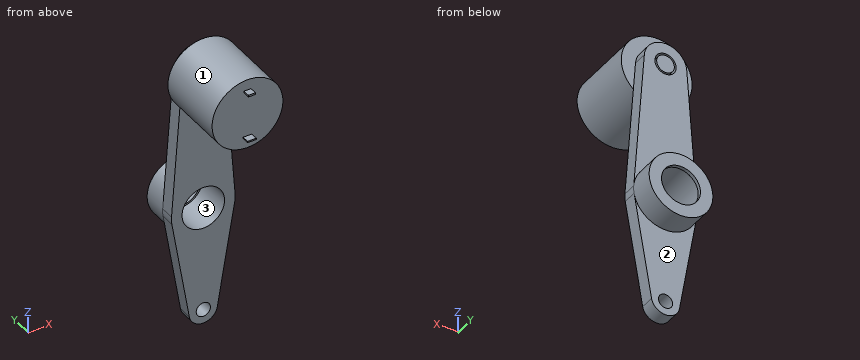
from build123d import *

# Parameters (mm, degrees)
EXTRUDE_1_DEPTH       = 4
SKETCH_3_R            = 9
EXTRUDE_2_DEPTH       = 7
SKETCH_4_R            = 3
CUT_EXTRUDE_1_DEPTH   = 48.391982444
SKETCH_5_R            = 6
CUT_EXTRUDE_2_DEPTH   = 10
SKETCH_7_R            = 5.5
CUT_EXTRUDE_3_DEPTH   = 49.145612469
HOLE_WIZARD_4_0_4_1_D = 4
SCALE1_SCALE          = 2
SKETCH1_R             = 20
EXTRUDE1_DEPTH        = 40
SKETCH2_R             = 5
EXTRUDE2_DEPTH        = 8
SKETCH3_W             = 4
SKETCH3_H             = 1
SKETCH3_W_2           = 4.944968004
SKETCH3_H_2           = 0.773994992
EXTRUDE3_DEPTH        = 4


with BuildPart() as part:
    # 草图1 → 凸台-拉伸1 (new body)
    with BuildSketch(Plane(origin=(0, 0, 0), x_dir=(1, 0, 0), z_dir=(0, 1, 0))):
        with BuildLine():
            Line((-8.974651804, -0.675), (-5.983101203, -40.45))
            ThreePointArc((-5.983101203, -40.45), (0, -46), (5.983101203, -40.45))
            Line((5.983101203, -40.45), (8.974651804, -0.675))
            ThreePointArc((8.974651804, -0.675), (8.990401386, 0.415551353), (8.874119675, 1.5))
            Line((8.874119675, 1.5), (3.944053189, 30.666666667))
            ThreePointArc((3.944053189, 30.666666667), (0, 34), (-3.944053189, 30.666666667))
            Line((-3.944053189, 30.666666667), (-8.874119675, 1.5))
            ThreePointArc((-8.874119675, 1.5), (-8.990401386, 0.415551353), (-8.974651804, -0.675))
        make_face()
    extrude(amount=EXTRUDE_1_DEPTH)

    # 草图3 → 凸台-拉伸2 (add)
    with BuildSketch(Plane(origin=(0, 4, 0), x_dir=(1, 0, 0), z_dir=(0, 1, 0))):
        with Locations(Location((0, 0, 0), (0, 0, 9.594068227))):
            Circle(SKETCH_3_R)
    extrude(amount=EXTRUDE_2_DEPTH)

    # 草图4 → 切除-拉伸1 (cut, through all)
    with BuildSketch(Plane(origin=(0, 4, 0), x_dir=(1, 0, 0), z_dir=(0, 1, 0))):
        with Locations(Location((0, -40, 0), (0, 0, 270))):
            Circle(SKETCH_4_R)
    extrude(amount=-CUT_EXTRUDE_1_DEPTH, mode=Mode.SUBTRACT)

    # 草图5 → 切除-拉伸2 (cut)
    with BuildSketch(Plane.XZ):
        with Locations(Location((0, 0, 0), (0, 0, 270))):
            Circle(SKETCH_5_R)
    extrude(amount=-CUT_EXTRUDE_2_DEPTH, mode=Mode.SUBTRACT)

    # 草图7 → 切除-拉伸3 (cut, through all)
    with BuildSketch(Plane(origin=(0, 11, 0), x_dir=(1, 0, 0), z_dir=(0, 1, 0))):
        with Locations(Location((0, 0, 0), (0, 0, 270))):
            Circle(SKETCH_7_R)
    extrude(amount=-CUT_EXTRUDE_3_DEPTH, mode=Mode.SUBTRACT)

    # Ø4.0 (4) 直径孔1 (through all)
    with Locations(Plane(origin=(0, 4, 0), x_dir=(1, 0, 0), z_dir=(0, 1, 0))):
        with Locations((0, 30)):
            Hole(HOLE_WIZARD_4_0_4_1_D / 2)


with BuildPart() as part_1:
    # Scale1: scaled about (0, 3.188915264, 5.875445323)
    add(part.part.scale(SCALE1_SCALE).moved(Location((0, -3.188915264, -5.875445323))))

    # Sketch1 → Extrude1 (add)
    with BuildSketch(Plane.XZ.offset(3.188915264)):
        with Locations(Location((0, 74.124554677, 0), (0, 0, 228.828880049))):
            Circle(SKETCH1_R)
    extrude(amount=EXTRUDE1_DEPTH)

    # Sketch2 → Extrude2 (add)
    with BuildSketch(Plane(origin=(0, -3.188915264, 0), x_dir=(1, 0, 0), z_dir=(0, 1, 0))):
        with Locations(Location((0, -74.124554677, 0), (0, 0, 90))):
            Circle(SKETCH2_R)
    extrude(amount=EXTRUDE2_DEPTH)

    # Sketch3 → Extrude3 (add)
    with BuildSketch(Plane.XZ.offset(43.188915264)):
        with Locations((0, 87.624554677)):
            Rectangle(SKETCH3_W, SKETCH3_H)
        with Locations((0, 60.737557181)):
            Rectangle(SKETCH3_W_2, SKETCH3_H_2)
    extrude(amount=EXTRUDE3_DEPTH)


solid = part_1.part
Model file for the job. Use its own axes, mm. Face numbers are marked on the shaded views. Round coordinates to 2 decimals unless told otherwise and drop trailing zeros. Order: outer loops, then holes, each group sorted by start corner. A loop starts at its lowest first (then second) coordinate and runs counter-clockwise, first axis right, second up. Notation, with made-up numbers: M 32,86.5 L 73,86.5 A20 cw 73,123.5 Z; hole C -13,28.5 d6. An arc over 180 degrees is marked long. Write each question's results on one line, items separated by ' | '. Start each with the question number.
(1) Saw through at D-D, the plane y = 9. Give the cut face in (x, z), then the cut area to 3 significant figures.
(2) Probe probe 1 along Y at (x, z) = (-3, -57.5); probe 2 along Y at (x, z) = (0.5, 60); probe 3 along X at (y, z) = (2, 3.5). List the from-to ranges inside material, lowest first. Write a range as from..to.
(3) Two-plate mould, pull along Z, no slides. Class the marked faces 1, 2 and 3: pulls with the +Z half, pulls with the -Z half, needs draft (parallel to the pull), parting line crosses it, or undercut.
(4) Drop flat-ended pins along their axis: pin 1 (12 mm diameter, centred on x = 4, z = -5, fed in from -Y); pin 2 (5 mm diameter, centred on x = 15, y = -22.5, fed in from -Z); pin 3 (1 mm diameter, centred on x = 3, z = 40.5, fed in from +Y); pin 4 (6 mm diameter, centred on x = -0.5, y = -35.5, fed in from -Z). Give the stop position or say it passes through.
(5) Saw through at B-B, the plane x = 0. State how many separate pieces and enclosed holes the cut face has, then the cut area to 3 significant figures.
(6) Saw through at C-C, the plane z = 3.5. Give the cut face in (x, y).
(7) Saw through at A-A, the plane y = 2. Give the cut face in (x, z).
Established:
1) outline: C 0,-5.88 d36; hole C 0,-5.88 d24 | area: 565 mm^2
2) probe 1: y = -3.19..4.81 | probe 2: y = -43.19..4.81 | probe 3: x = -17.35..-7.49, 7.49..17.35
3) face 1: parting line crosses it | face 2: needs draft | face 3: undercut
4) pin 1: passes through | pin 2: stops at z = 58.51 | pin 3: stops at y = 4.81 | pin 4: stops at z = 54.12
5) separate pieces: 3 | enclosed holes: 0 | area: 2,790 mm^2
6) outline: M -17.35,-3.19 L -7.49,-3.19 L -7.49,16.81 L -5.75,16.81 L -5.75,18.81 L -15.37,18.81 L -15.37,4.81 L -17.35,4.81 Z; M 5.75,16.81 L 7.49,16.81 L 7.49,-3.19 L 17.35,-3.19 L 17.35,4.81 L 15.37,4.81 L 15.37,18.81 L 5.75,18.81 Z
7) outline: M -17.95,-4.53 A18 ccw -17.75,-8.88 L -7.89,-67.21 A8 ccw 7.89,-67.21 L 17.75,-8.88 A18 ccw 17.95,-4.53 L 11.97,75.02 A12 ccw -11.97,75.02 Z; C 0,74.12 d10; hole C 0,-5.88 d24; hole C 0,74.12 d12; hole C 0,-65.88 d8
